For this review, use the dimensioned drawing (mm, ordinates from the lowest corner) and the shaded views. A direction names the side the tool comes from. Give positions to 0.01 mm unless a question says otherwise; leave off trailing zeros. Write each loop counter-clockwise with the first axis right and the second up, starting at its lowest first coordinate (ties: lowest second). Pieces come first, ordered by that corner, then holes. Notation, with made-up numbers: (-14.5, -20) -> (-9.5, -20) arc R32 ccw to (-9.5, 12) -> close; hole circle Ø5 at (-24, 6.25). An arc over 180 degrees is marked (long way). Return JSON: item names as keys, results as strings.
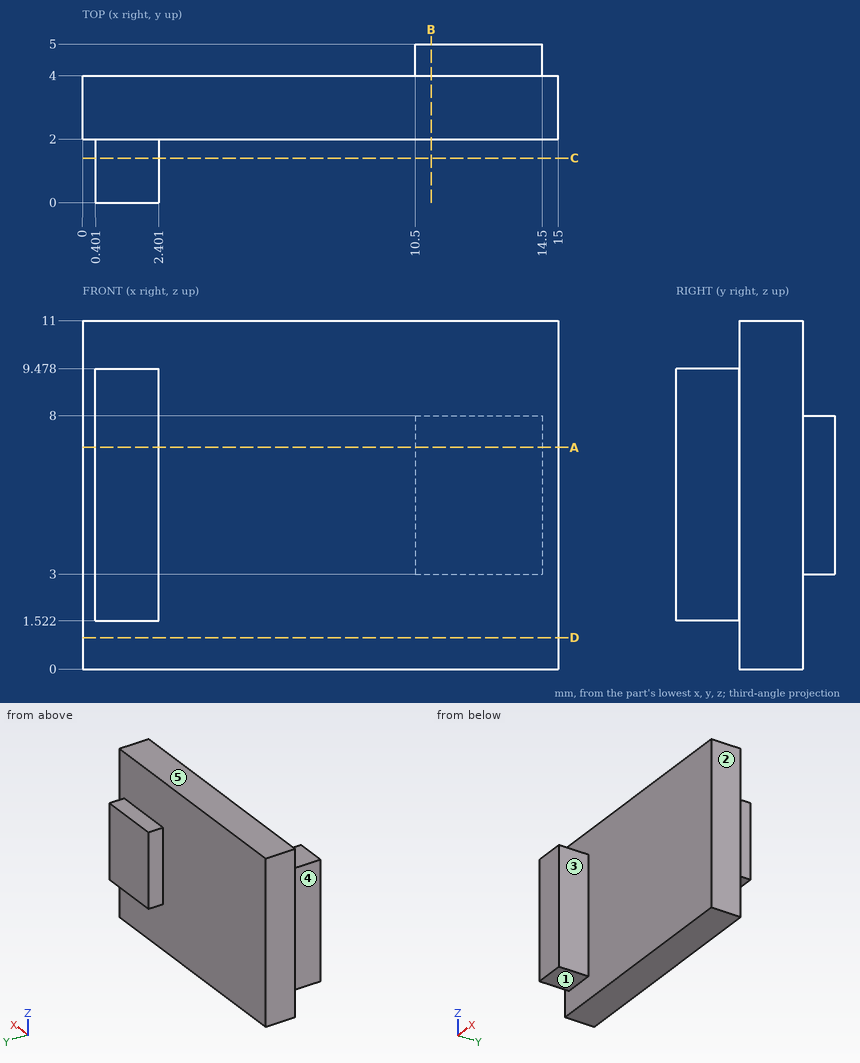
1. For the marked faces 1 and 2, list the 3-axis set-ups (+Z, -Z, +X, -X, +Y, -Y) from which the entire face can be reached by the end or side of a thin tool; tool diameter is ignored.
Results found:
{"face 1": "-Z, +X, -X, -Y", "face 2": "+Z, -Z, +X, +Y, -Y"}
2. To check wall thickness, follow probe 1 along Y at (x, z) = (9.25, 2); probe 2 along Y at (x, z) = (0.5, 2.5); probe 3 along X at (y, z) = (0.35, 4.25). State the ranges of each line that lie inside material, in increasing order.
Results found:
{"probe 1": "y = 2 to 4", "probe 2": "y = 0 to 4", "probe 3": "x = 0.4 to 2.4"}
3. Add section D-D, the plane z = 1. State the section outline as (x, y) points.
Results found:
{"outline": "(0, 2) -> (15, 2) -> (15, 4) -> (0, 4) -> close"}
4. Add section A-A, the plane z = 7. State the section outline as (x, y) points.
Results found:
{"outline": "(0, 2) -> (0.4, 2) -> (0.4, 0) -> (2.4, 0) -> (2.4, 2) -> (15, 2) -> (15, 4) -> (14.5, 4) -> (14.5, 5) -> (10.5, 5) -> (10.5, 4) -> (0, 4) -> close"}
5. Add section B-B, the plane x = 11. State the section outline as (y, z) points.
Results found:
{"outline": "(2, 0) -> (4, 0) -> (4, 3) -> (5, 3) -> (5, 8) -> (4, 8) -> (4, 11) -> (2, 11) -> close"}
6. Add section C-C, the plane y = 1.4. State the section outline as (x, z) points, plus the area to 3 significant figures.
Results found:
{"outline": "(0.4, 1.52) -> (2.4, 1.52) -> (2.4, 9.48) -> (0.4, 9.48) -> close", "area": "15.9 mm²"}
7. For pin 1 (0.5 mm diameter, centred on y = 4.5, z = 4.5, fed in from -X); pin 2 (0.6 mm diameter, centred on y = 0.5, z = 5.5, fed in from +X); pin 3 (3.5 mm diameter, centred on x = 6.5, z = 5.5, fed in from +Y), all flat-tipped, find the tip position at first contact; note any pin that passes through.
Results found:
{"pin 1": "stops at x = 10.5", "pin 2": "stops at x = 2.4", "pin 3": "stops at y = 4"}
8. The part is to be moulded in two halves that separate along X. For the marked faces 3, 4 and 5, say which applies: +X half, -X half, draft (parallel to the pull), parting line (faces both ways), or undercut.
Results found:
{"face 3": "+X half", "face 4": "-X half", "face 5": "draft"}
